from build123d import *

# Parameters (mm, degrees)
F0_W     = 151.2
F0_H     = 50
F1_DEPTH = 2.4
F0_H_2   = 98.8
F0_W_2   = 156
F0_H_3   = 156
F0_H_4   = 2.4
F2_DEPTH = 34
F3_R     = 20
F4_R     = 10


with BuildPart() as f1:
    # F0 (on Top) → F1 (new body)
    with BuildSketch(Plane.XY):
        with Locations((0, 50.6)):
            Rectangle(F0_W, F0_H)
    extrude(amount=F1_DEPTH)



with BuildPart() as f1b:
    # F0 (on Top) → F1, piece 2 (new body)
    with BuildSketch(Plane.XY):
        with Locations((0, -26.2)):
            Rectangle(F0_W, F0_H_2)
    extrude(amount=F1_DEPTH)


with BuildPart() as f1_1:
    add(f1.part)

    add(f1b.part)  # F2 merges F1b
    # F0 (on Top) → F2 (join)
    with BuildSketch(Plane.XY):
        Rectangle(F0_W_2, F0_H_3)
        Polygon((-75.6, 25.6), (-75.6, 75.6), (75.6, 75.6), (75.6, 25.6), (75.6, 23.2), (75.6, -75.6), (-75.6, -75.6), (-75.6, 23.2), align=None, mode=Mode.SUBTRACT)
        with Locations((0, 24.4)):
            Rectangle(F0_W, F0_H_4)
    extrude(amount=F2_DEPTH)

    # F3
    f3_edges = [f1_1.edges().sort_by_distance(p)[0] for p in [
        (0, -75.6, 2.4),
        (75.6, -26.2, 2.4),
        (0, 23.2, 2.4),
        (-75.6, -26.2, 2.4),
    ]]
    fillet(f3_edges, radius=F3_R)

    # F4
    f4_edges = [f1_1.edges().sort_by_distance(p)[0] for p in [
        (75.6, 50.6, 2.4),
        (-75.6, 50.6, 2.4),
    ]]
    fillet(f4_edges, radius=F4_R)


solid = f1_1.part
Could you check a few things on this model? Use its own coordinates, in mm. A direction names the side the tool comes from. Round coordinates to 2 decimals unless told otherwise and drop trailing zeros. Write each loop counter-clockwise with the first axis right and the second up, starting at its lowest first coordinate (ties: lowest second). Pieces come first, ordered by that corner, then holes. Notation, with made-up numbers: (89, 1) -> (124, 1) arc R35 cw to (124, 39) -> close; hole circle Ø11 at (73.5, -25). An arc over 180 degrees is marked (long way). Use a Markdown table: item, result.
1. If we section it at C-C (x = 10): List the corners of the cut face in (y, z) for me.
Answer key:
| item | result |
|---|---|
| outline | (-78, 0) -> (78, 0) -> (78, 34) -> (75.6, 34) -> (75.6, 2.4) -> (25.6, 2.4) -> (25.6, 34) -> (23.2, 34) -> (23.2, 22.4) arc R20 cw to (3.2, 2.4) -> (-55.6, 2.4) arc R20 cw to (-75.6, 22.4) -> (-75.6, 34) -> (-78, 34) -> close |
2. We'd pull the mould along Y, two halves only. Please class faces 3 (the face through (-1, 78, 17)), 4 (the face through (-75.6, -27, 28)), 5 (the face through (-1, 1, 0)): +Y half, -Y half, draft (parallel to the pull), parting line (faces both ways), or undercut.
Answer key:
| item | result |
|---|---|
| face 3 | +Y half |
| face 4 | undercut |
| face 5 | draft |
3. For pin 1 Ø10 at (x, y) = (32.5, -3.5) entering from +Z, with a flat end and sliding along its axis, tell me the tip position at first contact or that it passes through.
Answer key:
| item | result |
|---|---|
| pin 1 | stops at z = 2.4 |
4. Please list where these lines run through material, in increasing order: probe 1 along Y at (x, z) = (-40, 26); probe 2 along X at (y, z) = (-35.5, 29); probe 3 along Y at (x, z) = (33.5, 15.5).
Answer key:
| item | result |
|---|---|
| probe 1 | y = -78 to -75.6, 23.2 to 25.6, 75.6 to 78 |
| probe 2 | x = -78 to -75.6, 75.6 to 78 |
| probe 3 | y = -78 to -74.37, 21.97 to 25.6, 75.6 to 78 |
5. If we section it at B-B (y = 30): List the corners of the cut face in (x, z) for me, then the cut area to 3 significant figures.
Answer key:
| item | result |
|---|---|
| outline | (-78, 0) -> (78, 0) -> (78, 34) -> (75.6, 34) -> (75.6, 12.4) arc R10 cw to (65.6, 2.4) -> (-65.6, 2.4) arc R10 cw to (-75.6, 12.4) -> (-75.6, 34) -> (-78, 34) -> close |
| area | 569 mm^2 |
6. If we section it at A-A (z = 28.5): List the corners of the cut face in (x, y) for me, then the cut area to 3 significant figures.
Answer key:
| item | result |
|---|---|
| outline | (-78, -78) -> (78, -78) -> (78, 78) -> (-78, 78) -> close; hole (-75.6, -75.6) -> (75.6, -75.6) -> (75.6, 23.2) -> (-75.6, 23.2) -> close; hole (-75.6, 25.6) -> (75.6, 25.6) -> (75.6, 75.6) -> (-75.6, 75.6) -> close |
| area | 1,840 mm^2 |
7. If we section it at D-D (y = -60): List the corners of the cut face in (x, z) for me, then the cut area to 3 significant figures.
Answer key:
| item | result |
|---|---|
| outline | (-78, 0) -> (78, 0) -> (78, 34) -> (75.6, 34) -> (75.6, 22.4) arc R20 cw to (60, 2.89) -> (-60, 2.89) arc R20 cw to (-75.6, 22.4) -> (-75.6, 34) -> (-78, 34) -> close |
| area | 755 mm^2 |
8. Which directions (+Z, -Z, +X, -X, +Y, -Y) give clear straight access to the entire face, cutting with the end or side of a thin tool? Please do faces 1 (the face through (78, -1, 17)), 2 (the face through (-75.6, 50, 23)).
Answer key:
| item | result |
|---|---|
| face 1 | +Z, -Z, +X, +Y, -Y |
| face 2 | +Z |
